Input: part model. Units: mm. Frame: model coordinates. A direction names the side the tool comes from. Round coordinates to 2 decimals unless told otherwise and drop trailing zeros. Write each loop counter-clockwise with the first axis right and the second up, starting at its lowest first coordinate (ties: lowest second). Pieces come first, ordered by that corner, then holes. Notation, with made-up numbers: (74.25, 14) - (99.25, 14) arc R24 ccw to (99.25, 53) - close; hole circle Ø5 at (1, 21). An arc over 180 degrees is marked (long way). Use one line per item in the form item = value.
```python
from build123d import *

# Parameters (mm, degrees)
EXTRUDE_1_DEPTH     = 20
SKETCH_3_R          = 45
CUT_EXTRUDE_1_DEPTH = 302.784691461
SKETCH_4_R          = 55
CUT_EXTRUDE_2_DEPTH = 13
SKETCH_5_W          = 37.703420814
SKETCH_5_H          = 120
CUT_EXTRUDE_3_DEPTH = 5.4
CUT_EXTRUDE_4_DEPTH = 302.784691461
FILLET_1_R          = 5
CHAMFER_1_SIZE      = 5


with BuildPart() as part:
    # 草图2 → 凸台-拉伸1 (new body)
    with BuildSketch(Plane(origin=(0, 0, 0), x_dir=(1, 0, 0), z_dir=(0, 1, 0))):
        Polygon((0, 0), (135, 0), (135, -23), (265, -23), (265, -143), (135, -143), (135, -130), (0, -130), align=None)
    extrude(amount=EXTRUDE_1_DEPTH)

    # 草图3 → 切除-拉伸1 (cut, through all)
    with BuildSketch(Plane(origin=(0, 20, 0), x_dir=(1, 0, 0), z_dir=(0, 1, 0))):
        with Locations(Location((65, -65, 0), (0, 0, 270))):
            Circle(SKETCH_3_R)
    extrude(amount=-CUT_EXTRUDE_1_DEPTH, mode=Mode.SUBTRACT)

    # 草图4 → 切除-拉伸2 (cut)
    with BuildSketch(Plane(origin=(0, 20, 0), x_dir=(1, 0, 0), z_dir=(0, 1, 0))):
        with Locations(Location((65, -65, 0), (0, 0, 270))):
            Circle(SKETCH_4_R)
    extrude(amount=-CUT_EXTRUDE_2_DEPTH, mode=Mode.SUBTRACT)

    # 草图5 → 切除-拉伸3 (cut)
    with BuildSketch(Plane(origin=(0, 20, 0), x_dir=(1, 0, 0), z_dir=(0, 1, 0))):
        with Locations((200, -83)):
            Rectangle(SKETCH_5_W, SKETCH_5_H)
    extrude(amount=-CUT_EXTRUDE_3_DEPTH, mode=Mode.SUBTRACT)

    # 草图6 → 切除-拉伸4 (cut, through all)
    with BuildSketch(Plane(origin=(0, 20, 0), x_dir=(1, 0, 0), z_dir=(0, 1, 0))):
        with BuildLine():
            Line((157, -47.312507702), (157, -62.312507702))
            ThreePointArc((157, -62.312507702), (150, -69.312507702), (143, -62.312507702))
            Line((143, -62.312507702), (143, -47.312507702))
            ThreePointArc((143, -47.312507702), (150, -40.312507702), (157, -47.312507702))
        make_face()
        with BuildLine():
            Line((157, -105.55824709), (157, -120.55824709))
            ThreePointArc((157, -120.55824709), (150, -127.55824709), (143, -120.55824709))
            Line((143, -120.55824709), (143, -105.55824709))
            ThreePointArc((143, -105.55824709), (150, -98.55824709), (157, -105.55824709))
        make_face()
        with BuildLine():
            Line((257, -47.312507702), (257, -62.312507702))
            ThreePointArc((257, -62.312507702), (250, -69.312507702), (243, -62.312507702))
            Line((243, -62.312507702), (243, -47.312507702))
            ThreePointArc((243, -47.312507702), (250, -40.312507702), (257, -47.312507702))
        make_face()
        with BuildLine():
            Line((257, -105.55824709), (257, -120.55824709))
            ThreePointArc((257, -120.55824709), (250, -127.55824709), (243, -120.55824709))
            Line((243, -120.55824709), (243, -105.55824709))
            ThreePointArc((243, -105.55824709), (250, -98.55824709), (257, -105.55824709))
        make_face()
    extrude(amount=-CUT_EXTRUDE_4_DEPTH, mode=Mode.SUBTRACT)

    # 圆角1
    fillet_1_edges = [part.edges().sort_by_distance(p)[0] for p in [
        (135, 10, 23),
        (135, 10, 130),
    ]]
    fillet(fillet_1_edges, radius=FILLET_1_R)

    # 倒角1
    chamfer_1_edges = [part.edges().sort_by_distance(p)[0] for p in [
        (0, 10, 0),
        (135, 10, 0),
        (265, 10, 23),
        (265, 10, 143),
        (135, 10, 143),
        (0, 10, 130),
    ]]
    chamfer(chamfer_1_edges, length=CHAMFER_1_SIZE)


solid = part.part
```
(1) Cut plane B-B on x = 150. Output: boundary loops of the cut face in (y, z), then the cut area to 3 significant figures.
Derived:
outline = (0, 23) - (20, 23) - (20, 40.31) - (0, 40.31) - close; (0, 69.31) - (20, 69.31) - (20, 98.56) - (0, 98.56) - close; (0, 127.56) - (20, 127.56) - (20, 143) - (0, 143) - close
area = 1,240 mm^2
(2) First-contact query: pin 1 Ø0.9 at (y, z) = (13, 136) entering from -X; pin 2 Ø3 at (x, z) = (174.5, 123) entering from -Y; pin 3 Ø1 at (x, z) = (103, 94.5) entering from +Y. Flat tips, straight axial feed; report the tip coordinate or a pass-through.
Derived:
pin_1 = 135
pin_2 = 0
pin_3 = 7
(3) Cut plane A-A on x = 65. Output: boundary loops of the cut face in (y, z), then the cut area to 3 significant figures.
Derived:
outline = (0, 0) - (20, 0) - (20, 10) - (7, 10) - (7, 20) - (0, 20) - close; (0, 110) - (7, 110) - (7, 120) - (20, 120) - (20, 130) - (0, 130) - close
area = 540 mm^2
(4) Draft query along X for faces 4 (the face through (262, 10, 141)), 5 (the face through (68, 10, 130)), 6 (the face through (200, 14.6, 82)), 7 (the face through (3, 10, 128)). Return one class per face: released by +X, released by -X, zero draft, split by the parting line, or undercut.
Derived:
face_4 = released by +X
face_5 = zero draft
face_6 = undercut
face_7 = released by -X
(5) Access query for faces 1 (the face through (243, 10, 113)), 2 (the face through (181.148, 17, 84)), 3 (the face through (67.418, 13.591, 10.053)). Directions: +Z, -Z, +X, -X, +Y, -Y. A direction counts if a zero-diameter tool reaches every point of the face in a straight line with its end or side. Return the directions, or none.
Derived:
face_1 = +Y, -Y
face_2 = +Z, -Z, +Y
face_3 = +Y
(6) Cut plane D-D on z = 25.5. Output: boundary loops of the cut face in (x, y).
Derived:
outline = (0, 0) - (43.44, 0) - (43.44, 7) - (26.73, 7) - (26.73, 20) - (0, 20) - close; (86.56, 0) - (262.5, 0) - (262.5, 20) - (218.85, 20) - (218.85, 14.6) - (181.15, 14.6) - (181.15, 20) - (103.27, 20) - (103.27, 7) - (86.56, 7) - close
(7) Material intervals for L1, parallel to X at y = 5, z = 65; L2, parallel to X at y = 17, z = 81.5; L3, parallel to Z at x = 249, y = 5.75, sorted ascending.
Derived:
L1 = 0 to 20, 110 to 143.54, 156.46 to 243.54, 256.46 to 265
L2 = 0 to 12.53, 117.47 to 181.15, 218.85 to 265
L3 = 23 to 40.38, 69.24 to 98.63, 127.49 to 143
(8) Cut plane C-C on z = 112.5. Output: boundary loops of the cut face in (x, y).
Derived:
outline = (0, 0) - (143, 0) - (143, 20) - (92.73, 20) - (92.73, 7) - (37.27, 7) - (37.27, 20) - (0, 20) - close; (157, 0) - (243, 0) - (243, 20) - (218.85, 20) - (218.85, 14.6) - (181.15, 14.6) - (181.15, 20) - (157, 20) - close; (257, 0) - (265, 0) - (265, 20) - (257, 20) - close
